Verification items for the finished model (mm, model axes). Face numbers are marked on the shaded views. A direction names the side the tool comes from. Round coordinates to 2 decimals unless told otherwise and drop trailing zeros. Write each loop counter-clockwise with the first axis right and the second up, starting at its lowest first coordinate (ties: lowest second). Pieces come first, ordered by that corner, then holes. Notation, with made-up numbers: (-7, 10.25) - (8, 10.25) arc R30 cw to (8, 48.25) - close; hole circle Ø2 at (7.25, 53). An arc over 180 degrees is marked (long way). Answer as a JSON object with one key per item and string values. Group by question number.
1) Thickness scan on line 1 (X direction, y = -0.5, z = -4.25); line 2 (Z direction, x = -23, y = -0.25); line 3 (Y direction, x = 3, z = 2.5). Record the ranges inside material, lowest first.
2) Section check A-A (x = 24). Enter the section's corners in (y, z) (3 decimals).
3) Go/stop test with flat-tipped pins: pin 1 Ø5 at (x, y) = (9, 3) entering from +Z; pin 2 Ø1 at (y, z) = (-1, -4) entering from +X; pin 3 Ø2 at (x, z) = (8.5, 2.5) entering from +Y. Record where each tip stops, or that it passes through.
4) Set-up check for the marked faces 1 and 2: record each of +Z, -Z, +X, -X, +Y, -Y from which the full face is reachable in a straight line by a thin tool's end or side.
```python
from build123d import *

# Parameters (mm, degrees)
SKETCH5_R           = 3.175
BOSS_EXTRUDE3_DEPTH = 50.8
CHAMFER1_SIZE       = 0.9525
BOSS_EXTRUDE4_DEPTH = 4.365625
SKETCH8_OUTSIDE_W   = 221.468
SKETCH8_OUTSIDE_H   = 223.188
SKETCH8_OUTSIDE_R   = 5.55625
CUT_EXTRUDE3_DEPTH  = 56.814699209
CUT_EXTRUDE3_DRAFT  = -60


with BuildPart() as part:
    # Sketch5 → Boss-Extrude3 (new body)
    with BuildSketch(Plane(origin=(27.5828125, 0, 0), x_dir=(0, 0, -1), z_dir=(1, 0, 0))):
        Circle(SKETCH5_R)
    extrude(amount=-BOSS_EXTRUDE3_DEPTH)

    # Chamfer1
    chamfer1_edges = [part.edges().sort_by_distance(p)[0] for p in [
        (27.5828125, 0, 3.175),
    ]]
    chamfer(chamfer1_edges, length=CHAMFER1_SIZE)

    # Sketch11 → Revolve1 (revolve)
    with BuildSketch(Plane.XY):
        Polygon((-23.2171875, 3.175), (-23.2171875, 0), (11.7078125, 0), (8.5328125, 3.175), align=None)
    revolve(axis=Axis((-23.2171875, 0, 0), (1, 0, 0)))

    # Sketch6 → Boss-Extrude4 (add)
    with BuildSketch(Plane.ZY.offset(23.2171875)):
        Polygon((5.55625, 3.207902433), (0, 6.415804866), (-5.55625, 3.207902433), (-5.55625, -3.207902433), (0, -6.415804866), (5.55625, -3.207902433), align=None)
    extrude(amount=BOSS_EXTRUDE4_DEPTH)


with BuildPart() as cut_extrude3_tool:
    # Sketch8 outside → Cut-Extrude3 (with draft: the straight prism first)
    with BuildSketch(Plane.ZY.offset(27.5828125)):
        Rectangle(SKETCH8_OUTSIDE_W, SKETCH8_OUTSIDE_H)
        Circle(SKETCH8_OUTSIDE_R, mode=Mode.SUBTRACT)
    extrude(amount=-CUT_EXTRUDE3_DEPTH)
    # Cut-Extrude3: the draft: its side faces are tilted about the plane it starts from
    cut_extrude3_sides = [cut_extrude3_tool.faces().sort_by_distance(p)[0] for p in [
        (0.824537104, -111.594, 0),
        (0.824537104, 0, 110.734),
        (0.824537104, 111.594, 0),
        (0.824537104, 0, -110.734),
        (0.824537104, 0, -5.55625),
    ]]
    draft(cut_extrude3_sides, Plane.ZY.offset(27.5828125), CUT_EXTRUDE3_DRAFT)


with BuildPart() as part_1:
    add(part.part)

    # Cut-Extrude3: cut by cut_extrude3_tool
    add(cut_extrude3_tool.part, mode=Mode.SUBTRACT)


solid = part_1.part
```
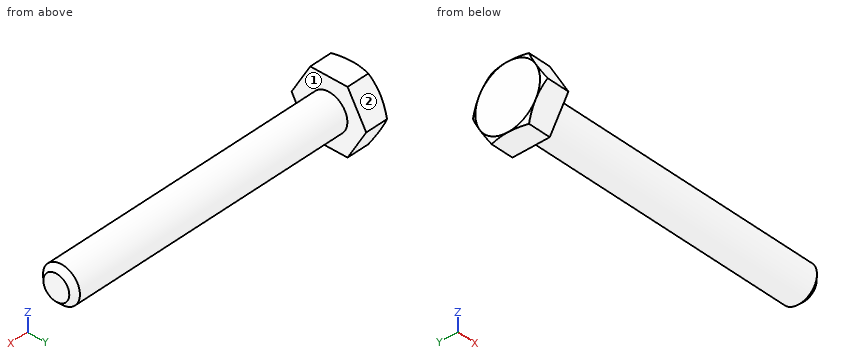
Returned:
{
 "1": {"line 1": "-27.58 to -23.22", "line 2": "-3.17 to 3.17", "line 3": "-1.96 to 1.96"},
 "2": {"outline": "circle Ø6.35 at (0, 0)"},
 "3": {"pin 1": "z = 3.14", "pin 2": "x = -23.22", "pin 3": "y = 2.8"},
 "4": {"face 1": "+X", "face 2": "+Z, +X, -X, +Y"}
}
